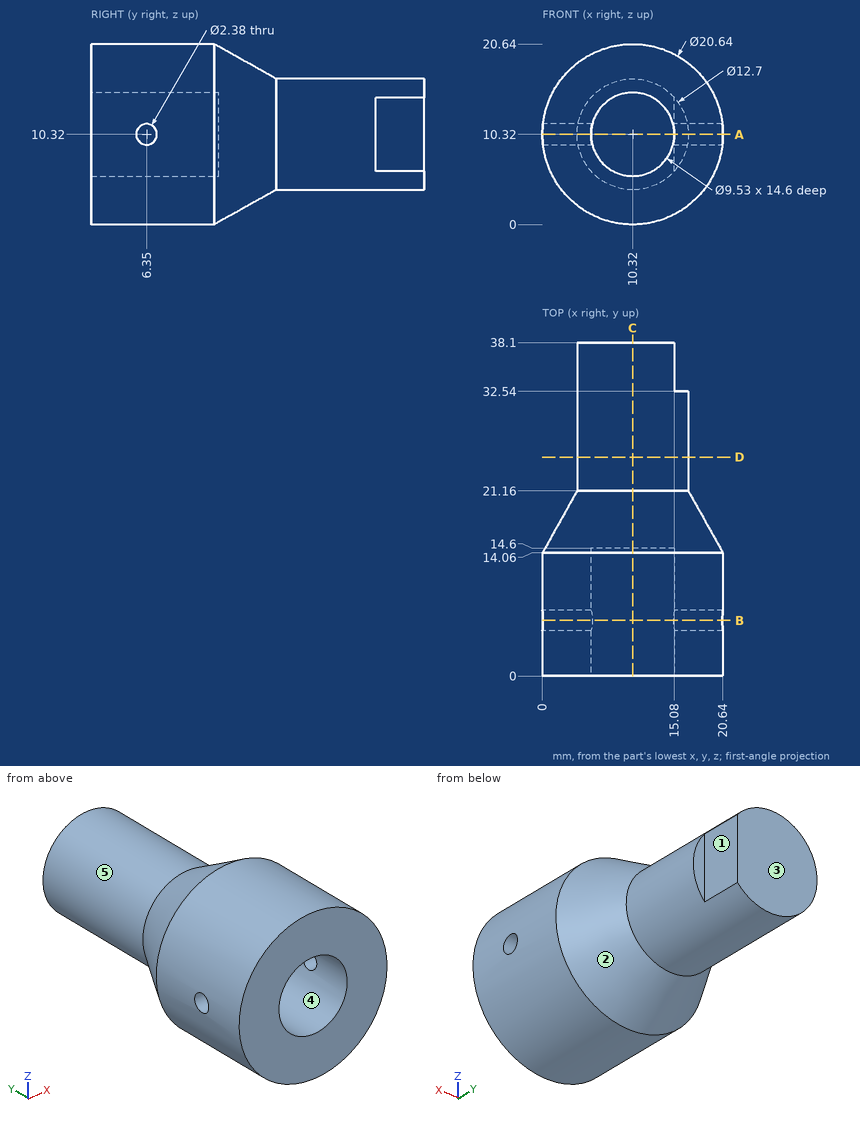
Input: dimensioned drawing with shaded views. Units: mm. Origin: part minimum x, y, z. A direction names the side the tool comes from. Give positions to 0.01 mm unless a question says otherwise; leave off trailing zeros. Write each loop counter-clockwise with the first axis right and the second up, starting at its lowest first coordinate (ties: lowest second). Pieces come first, ordered by that corner, then holes. Notation, with made-up numbers: M -17.75,47 L 32.25,47 A29 cw 32.25,76 Z; hole C 47,71 d5. An arc over 180 degrees is marked long. Return JSON: item names as keys, results as strings. Group by question number.
1) Material intervals for line 1 along X through (y, z) = (3.5, 10.32) (3 decimals); line 2 along Z through (x, y) = (11, 9); line 3 along Z through (x, y) = (6, 3), sorted ascending. Write a range as [from, to].
2) Pull-direction query (Z, two-part tool) for the marked faces 3, 4 and 5; classes: pulls with the +Z half, pulls with the -Z half, needs draft (parallel to the pull), parting line crosses it, or undercut.
3) Cut plane B-B, the plane y = 6.35. Output: boundary loops of the cut face in (x, z) (3 decimals).
4) Pin query (flat end, axial travel): P1, Ø10, axis at x = 6, z = 12, coming from the -Y side; P2, Ø10, axis at x = 15.5, y = 25.5, coming from the +Z side; P3, Ø5, axis at y = 31.5, z = 9, coming from the +X side; P4, Ø2, axis at y = 5, z = 15.5, coming from the +X side. Return the tip coordinate at first contact, or that it passes through.
5) Cut plane A-A, the plane z = 10.32. Output: boundary loops of the cut face in (x, y) (3 decimals), plus the area to 3 significant figures.
6) Set-up query: the marked faces 1 and 2. Return all of +Z, -Z, +X, -X, +Y, -Y with unobstructed straight access to the full face (end or side cutting, diameter ignored); none if empty.
7) Cut plane C-C, the plane x = 10.32. Output: boundary loops of the cut face in (y, z) (3 decimals), plus the area to 3 significant figures.
8) Cut plane D-D, the plane y = 25. Output: boundary loops of the cut face in (x, z), plus the area to 3 significant figures.
Recorded:
{
 "1": {"line 1": "x = [0, 5.555], [15.085, 20.64]", "line 2": "z = [0.02, 5.6], [15.04, 20.62]", "line 3": "z = [0.95, 8.31], [12.33, 19.69]"},
 "2": {"face 3": "needs draft", "face 4": "undercut", "face 5": "parting line crosses it"},
 "3": {"outline": "M 0.069,9.13 A10.32 ccw 20.571,9.13 L 14.934,9.13 A4.765 cw 5.706,9.13 Z; M 0.069,11.51 L 5.706,11.51 A4.765 cw 14.934,11.51 L 20.571,11.51 A10.32 ccw Z"},
 "4": {"P1": "stops at y = 0", "P2": "stops at z = 16.67", "P3": "stops at x = 16.67", "P4": "stops at x = 19.76"},
 "5": {"outline": "M 0,0 L 5.555,0 L 5.555,5.16 L 0,5.16 Z; M 0,7.54 L 5.555,7.54 L 5.555,14.6 L 15.085,14.6 L 15.085,7.54 L 20.64,7.54 L 20.64,14.06 L 16.67,21.16 L 16.67,32.54 L 15.08,32.54 L 15.08,38.1 L 3.97,38.1 L 3.97,21.16 L 0,14.06 Z; M 15.085,0 L 20.64,0 L 20.64,5.16 L 15.085,5.16 Z", "area": "449 mm²"},
 "6": {"face 1": "+Z, -Z, +X, +Y", "face 2": "+Y"},
 "7": {"outline": "M 0,0 L 14.06,0 L 21.16,3.97 L 38.1,3.97 L 38.1,16.67 L 21.16,16.67 L 14.06,20.64 L 0,20.64 L 0,15.085 L 14.6,15.085 L 14.6,5.555 L 0,5.555 Z", "area": "485 mm²"},
 "8": {"outline": "C 10.32,10.32 d12.7", "area": "127 mm²"}
}
